Check sheet for the modelled part. Datum: model origin and axes. Units: mm. Give positions to 0.01 mm unless a question says otherwise; leave off trailing zeros. Order: outer loops, then holes, each group sorted by start corner. A loop starts at its lowest first (then second) coordinate and runs counter-clockwise, first axis right, second up.
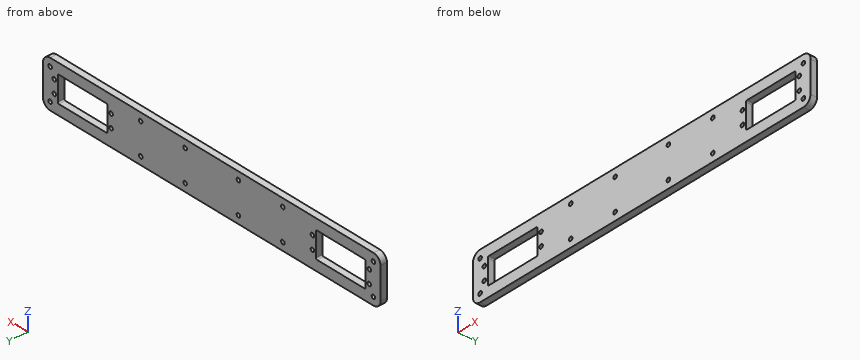
from build123d import *

# Parameters (mm, degrees)
SKETCH1_W           = 285
SKETCH1_H           = 36
SKETCH1_R           = 1.5
SKETCH1_W_2         = 42
SKETCH1_H_2         = 20
BOSS_EXTRUDE2_DEPTH = 5
FILLET1_R           = 6
FILLET2_R           = 1


with BuildPart() as part:
    # Sketch1 → Boss-Extrude2 (new body)
    with BuildSketch(Plane(origin=(0, 0, 0), x_dir=(1, 0, 0), z_dir=(0, 1, 0))):
        Rectangle(SKETCH1_W, SKETCH1_H)
        with Locations(Location((-85, -5, 0), (0, 0, 270))):
            Circle(SKETCH1_R, mode=Mode.SUBTRACT)
        with Locations(Location((-85, 5, 0), (0, 0, 270))):
            Circle(SKETCH1_R, mode=Mode.SUBTRACT)
        with Locations(Location((-133, 5, 0), (0, 0, 270))):
            Circle(SKETCH1_R, mode=Mode.SUBTRACT)
        with Locations(Location((-133, -5, 0), (0, 0, 270))):
            Circle(SKETCH1_R, mode=Mode.SUBTRACT)
        with Locations(Location((133, -5, 0), (0, 0, 90))):
            Circle(SKETCH1_R, mode=Mode.SUBTRACT)
        with Locations(Location((133, 5, 0), (0, 0, 90))):
            Circle(SKETCH1_R, mode=Mode.SUBTRACT)
        with Locations(Location((85, -5, 0), (0, 0, 90))):
            Circle(SKETCH1_R, mode=Mode.SUBTRACT)
        with Locations(Location((85, 5, 0), (0, 0, 90))):
            Circle(SKETCH1_R, mode=Mode.SUBTRACT)
        with Locations(Location((-22.5, -12, 0), (0, 0, 270))):
            Circle(SKETCH1_R, mode=Mode.SUBTRACT)
        with Locations(Location((-22.5, 12, 0), (0, 0, 90))):
            Circle(SKETCH1_R, mode=Mode.SUBTRACT)
        with Locations(Location((-136.5, -12, 0), (0, 0, 270))):
            Circle(SKETCH1_R, mode=Mode.SUBTRACT)
        with Locations(Location((-136.5, 12, 0), (0, 0, 90))):
            Circle(SKETCH1_R, mode=Mode.SUBTRACT)
        with Locations(Location((22.5, -12, 0), (0, 0, 90))):
            Circle(SKETCH1_R, mode=Mode.SUBTRACT)
        with Locations(Location((22.5, 12, 0), (0, 0, 270))):
            Circle(SKETCH1_R, mode=Mode.SUBTRACT)
        with Locations(Location((136.5, -12, 0), (0, 0, 90))):
            Circle(SKETCH1_R, mode=Mode.SUBTRACT)
        with Locations(Location((136.5, 12, 0), (0, 0, 270))):
            Circle(SKETCH1_R, mode=Mode.SUBTRACT)
        with Locations(Location((-60, 12, 0), (0, 0, 270))):
            Circle(SKETCH1_R, mode=Mode.SUBTRACT)
        with Locations(Location((-60, -12, 0), (0, 0, 90))):
            Circle(SKETCH1_R, mode=Mode.SUBTRACT)
        with Locations(Location((60, -12, 0), (0, 0, 270))):
            Circle(SKETCH1_R, mode=Mode.SUBTRACT)
        with Locations(Location((60, 12, 0), (0, 0, 90))):
            Circle(SKETCH1_R, mode=Mode.SUBTRACT)
        with Locations((-109, 0)):
            Rectangle(SKETCH1_W_2, SKETCH1_H_2, mode=Mode.SUBTRACT)
        with Locations((109, 0)):
            Rectangle(SKETCH1_W_2, SKETCH1_H_2, mode=Mode.SUBTRACT)
    extrude(amount=BOSS_EXTRUDE2_DEPTH)

    # Fillet1
    fillet1_edges = [part.edges().sort_by_distance(p)[0] for p in [
        (142.5, 2.5, 18),
        (-142.5, 2.5, 18),
        (-142.5, 2.5, -18),
        (142.5, 2.5, -18),
    ]]
    fillet(fillet1_edges, radius=FILLET1_R)

    # Fillet2
    fillet2_edges = [part.edges().sort_by_distance(p)[0] for p in [
        (-88, 2.5, 10),
        (-88, 2.5, -10),
        (-130, 2.5, -10),
        (-130, 2.5, 10),
        (130, 2.5, -10),
        (88, 2.5, -10),
        (88, 2.5, 10),
        (130, 2.5, 10),
    ]]
    fillet(fillet2_edges, radius=FILLET2_R)


solid = part.part
1) Material ranges on L1, parallel to Z at x = -133, y = 1.3; L2, parallel to X at y = 1.45, z = -0.5; L3, parallel to Z at x = -117, y = 1.55, recorded low to high.
Recorded:
L1: z = -18 to -6.5, -3.5 to 3.5, 6.5 to 18
L2: x = -142.5 to -130, -88 to 88, 130 to 142.5
L3: z = -18 to -10, 10 to 18
2) Section check B-B, the plane x = -110. Record the cut outline in (y, z).
Recorded:
outline: (0, -18) - (5, -18) - (5, -10) - (0, -10) - close; (0, 10) - (5, 10) - (5, 18) - (0, 18) - close
3) Depth check by flat-ended pin: pin 1 Ø2.5 at (x, z) = (133, -5) entering from +Y. Enter the tip coordinate at first touch or a pass-through.
Recorded:
pin 1: passes through
4) Section check A-A, the plane z = 0. Record the cut outline in (x, y).
Recorded:
outline: (-142.5, 0) - (-130, 0) - (-130, 5) - (-142.5, 5) - close; (-88, 0) - (88, 0) - (88, 5) - (-88, 5) - close; (130, 0) - (142.5, 0) - (142.5, 5) - (130, 5) - close
5) Section check C-C, the plane y = 3.5. State how many separate pieces and enclosed holes the cut face has, then the cut area to 3 significant figures.
Recorded:
separate pieces: 1
enclosed holes: 22
area: 8,410 mm2
